Work out the finished part from the listing and answer in its coordinate system (mm). Give positions to 0.01 mm unless a question says otherwise; leave off trailing zeros. Loops run counter-clockwise (first coordinate to the right, second up) from the corner with the lowest first, then second, coordinate; pieces in that order, holes last. Notation, with made-up numbers: (24, -15.75) - (78, -15.75) arc R17 cw to (78, -11.75) - close; hole circle Ø8 at (43, 73.5). An arc over 180 degrees is marked (long way). Use CSV: the item, a comma, the result in double quotes.
from build123d import *

# Parameters (mm, degrees)
BOSS_EXTRUDE1_DEPTH = 5.08
CUT_EXTRUDE1_DEPTH  = 2.54
SKETCH5_R           = 1.5621
CUT_EXTRUDE2_DEPTH  = 133.476280518
SKETCH2_R           = 3.2512
CUT_EXTRUDE3_DEPTH  = 133.476280518


with BuildPart() as part:
    # Sketch1 → Boss-Extrude1 (new body)
    with BuildSketch(Plane.XY):
        with BuildLine():
            Line((0, 8.89), (123.19, 8.89))
            ThreePointArc((123.19, 8.89), (132.08, 0), (123.19, -8.89))
            Line((123.19, -8.89), (0, -8.89))
            ThreePointArc((0, -8.89), (-8.89, 0), (0, 8.89))
        make_face()
    extrude(amount=BOSS_EXTRUDE1_DEPTH)

    # Sketch4 → Cut-Extrude1 (cut)
    with BuildSketch(Plane(origin=(0, 0, 0), x_dir=(-1, 0, 0), z_dir=(0, 0, -1))):
        with BuildLine():
            Line((-5.600440074, 4.064037393), (-16.637267213, 2.893836949))
            ThreePointArc((-16.637267213, 2.893836949), (-19.240499434, -0.001815049), (-16.63365711, -2.89421744))
            Line((-16.63365711, -2.89421744), (-5.349174405, -4.076443038))
            ThreePointArc((-5.349174405, -4.076443038), (-4.669876023, -4.256197229), (-4.077266325, -4.633783784))
            ThreePointArc((-4.077266325, -4.633783784), (0, -6.1722), (4.077266325, -4.633783784))
            ThreePointArc((4.077266325, -4.633783784), (4.669876023, -4.256197229), (5.349174405, -4.076443038))
            Line((5.349174405, -4.076443038), (16.63365711, -2.89421744))
            ThreePointArc((16.63365711, -2.89421744), (19.2405, 0), (16.63365711, 2.89421744))
            Line((16.63365711, 2.89421744), (5.349174405, 4.076443038))
            ThreePointArc((5.349174405, 4.076443038), (4.669876023, 4.256197229), (4.077266325, 4.633783784))
            ThreePointArc((4.077266325, 4.633783784), (0, 6.1722), (-4.077266325, 4.633783784))
            ThreePointArc((-4.077266325, 4.633783784), (-4.786476333, 4.20888501), (-5.600440074, 4.064037393))
        make_face()
    extrude(amount=-CUT_EXTRUDE1_DEPTH, mode=Mode.SUBTRACT)

    # Sketch5 → Cut-Extrude2 (cut, through all)
    with BuildSketch(Plane.XY.offset(5.08)):
        Circle(SKETCH5_R)
    extrude(amount=-CUT_EXTRUDE2_DEPTH, mode=Mode.SUBTRACT)

    # Sketch2 → Cut-Extrude3 (cut, through all)
    with BuildSketch(Plane(origin=(0, 0, 0), x_dir=(-1, 0, 0), z_dir=(0, 0, -1))):
        with Locations((-123.19, 0)):
            Circle(SKETCH2_R)
    extrude(amount=-CUT_EXTRUDE3_DEPTH, mode=Mode.SUBTRACT)


solid = part.part
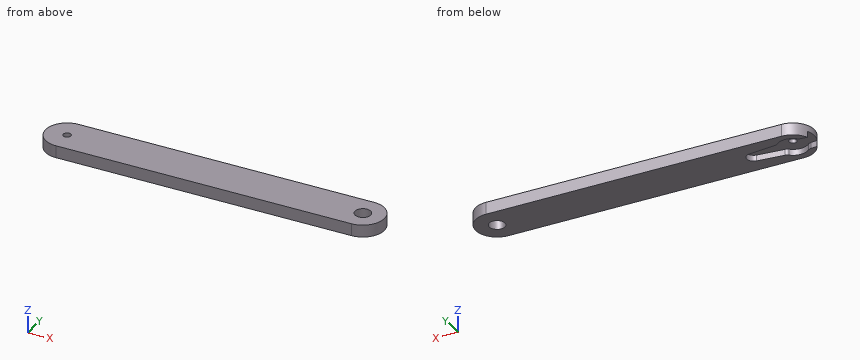
Item 1: Find the intervals of material crossed by line 1 (X direction, y = -0.25, z = 2.35); line 2 (Z direction, x = 0.5, y = 5); line 3 (X direction, y = -2, z = 3.85), in increasing order.
Determined:
line 1,"x = 19.23 to 119.95, 126.43 to 132.08"
line 2,"z = 2.54 to 5.08"
line 3,"x = -8.66 to 120.63, 125.75 to 131.85"
Item 2: Given P1, Ø3, axis at y = -5.5, z = 2, coming from the +X side; P2, Ø3, axis at y = -3.5, z = 1, coming from the -X side; P3, Ø4, axis at x = 123.19, y = 0, coming from the +Z side, each flat-ended and moving along its own axis, determine where each tip first touches the part or whether it passes through.
Determined:
P1,"stops at x = 131.13"
P2,"stops at x = -8.04"
P3,"passes through"
Item 3: A cutting plane is placed at A-A on y = 0. Determine the outline of the cut face in (x, z), and give its area (3 significant figures).
Determined:
outline,"(-8.89, 2.54) - (-1.56, 2.54) - (-1.56, 5.08) - (-8.89, 5.08) - close; (1.56, 2.54) - (19.24, 2.54) - (19.24, 0) - (119.94, 0) - (119.94, 5.08) - (1.56, 5.08) - close; (126.44, 0) - (132.08, 0) - (132.08, 5.08) - (126.44, 5.08) - close"
area,"604 mm²"
Item 4: A cutting plane is placed at B-B on z = 1.7. Determine the outline of the cut face in (x, y).
Determined:
outline,"(-8.04, -3.79) arc R8.89 ccw to (0, -8.89) - (123.19, -8.89) arc R8.89 ccw to (123.19, 8.89) - (0, 8.89) arc R8.89 ccw to (-8.04, 3.79) - (-5.35, 4.08) arc R2.29 ccw to (-4.08, 4.63) arc R6.17 cw to (4.08, 4.63) arc R2.29 ccw to (5.6, 4.06) - (16.64, 2.89) arc R2.91 cw to (16.63, -2.89) - (5.35, -4.08) arc R2.29 ccw to (4.08, -4.63) arc R6.17 cw to (-4.08, -4.63) arc R2.29 ccw to (-5.35, -4.08) - close; hole circle Ø6.5 at (123.19, 0)"
